Build history of the part. All positions in model axes, mm. Coordinates: 2 decimals unless noted, no trailing zeros. Loops run counter-clockwise (first coordinate to the right, second up) from the corner with the lowest first, then second, coordinate; pieces in that order, holes last.
Item 1: Drill centre lines: line 1 along Z through (x, y) = (-191, 0.7); line 2 along X through (y, z) = (3.2, 124). Where is each one in solid material? Low to high.
Item 2: Flat gauge pins, fed straight in: pin 1 (1.5 mm diameter, centred on y = 2, z = 132.5, fed in from +X); pin 2 (2.5 mm diameter, centred on y = 2, z = 148.5, fed in from -X). Where does each tip first touch, or does it go through?
Item 3: Cut at A-A (x = -209). List the corners of the cut face in (y, z), and give its area (3 significant figures).
Item 4: Cut at C-C (z = -139). List the corners of the cut face in (x, y), and give its area (4 significant figures).
Item 5: Cut at B-B (y = 1.65). List the corners of the cut face in (x, z), and give its area (3 significant figures).
from build123d import *

# Parameters (mm, degrees)
SKETCH1_W           = 500
SKETCH1_H           = 500
BOSS_EXTRUDE1_DEPTH = 5
CUT_EXTRUDE1_DEPTH  = 5


with BuildPart() as part:
    # Sketch1 → Boss-Extrude1 (new body)
    with BuildSketch(Plane(origin=(0, 0, 0), x_dir=(1, 0, 0), z_dir=(0, 1, 0))):
        Rectangle(SKETCH1_W, SKETCH1_H)
    extrude(amount=BOSS_EXTRUDE1_DEPTH)

    # Sketch3 → Cut-Extrude1 (cut)
    with BuildSketch(Plane(origin=(0, 5, 0), x_dir=(1, 0, 0), z_dir=(0, 1, 0))):
        Polygon((-187.5, 205), (-250, 205), (-250, 155), (-250, 105), (-187.5, 105), align=None)
        Polygon((-187.5, -105), (-250, -105), (-250, -155), (-250, -205), (-187.5, -205), align=None)
        Polygon((250, -155), (250, -105), (187.5, -105), (187.5, -205), (250, -205), align=None)
        Polygon((250, 155), (250, 205), (187.5, 205), (187.5, 105), (250, 105), align=None)
    extrude(amount=-CUT_EXTRUDE1_DEPTH, mode=Mode.SUBTRACT)


solid = part.part
Filled sheet:
1. line 1: z = -250 to -205, -105 to 105, 205 to 250
1. line 2: x = -187.5 to 187.5
2. pin 1: stops at x = 187.5
2. pin 2: stops at x = -187.5
3. outline: (0, -250) - (5, -250) - (5, -205) - (0, -205) - close; (0, -105) - (5, -105) - (5, 105) - (0, 105) - close; (0, 205) - (5, 205) - (5, 250) - (0, 250) - close
3. area: 1,500 mm2
4. outline: (-187.5, 0) - (187.5, 0) - (187.5, 5) - (-187.5, 5) - close
4. area: 1,875 mm2
5. outline: (-250, -250) - (250, -250) - (250, -205) - (187.5, -205) - (187.5, -105) - (250, -105) - (250, 105) - (187.5, 105) - (187.5, 205) - (250, 205) - (250, 250) - (-250, 250) - (-250, 205) - (-187.5, 205) - (-187.5, 105) - (-250, 105) - (-250, -105) - (-187.5, -105) - (-187.5, -205) - (-250, -205) - close
5. area: 225,000 mm2
